Drawing for the job (mm, zero at the part's lowest x, y, z). Coordinates: 2 decimals unless noted, no trailing zeros. Write each loop counter-clockwise with the first axis right and the second up, starting at its lowest first coordinate (ties: lowest second). Pieces come first, ordered by that corner, then holes. Notation, with made-up numbers: M 44.25,13 L 92.25,13 A22 cw 92.25,45 Z; hole C 28.5,23 d9. An arc over 180 degrees is marked long. Put each result on its own line as item: value. Start each with the question number.
Q1. Drop flat-ended pins along their axis: pin 1 (5 mm diameter, centred on x = 25, y = 4.5, fed in from +Z); pin 2 (3 mm diameter, centred on x = 41, y = 6.5, fed in from -Z); pin 3 (3 mm diameter, centred on y = 4.5, z = 2, fed in from +X). Give the stop position or say it passes through.
Q2. Cut at D-D (x = 19.5). Write the cut outline in (y, z), then the cut area to 3 significant figures.
Q3. Cut at A-A (x = 37.5). Write the cut outline in (y, z), then the cut area to 3 significant figures.
Q4. Cut at C-C (z = 0.5). Write the cut outline in (x, y).
Q5. Drill centre lines: line 1 along X through (y, z) = (3, 3.25); line 2 along Z through (x, y) = (33.5, 9.75); line 3 along X through (y, z) = (9.25, 6). Where is each one in solid material? Low to high.
Q6. Cut at B-B (y = 9). Write the cut outline in (x, z).
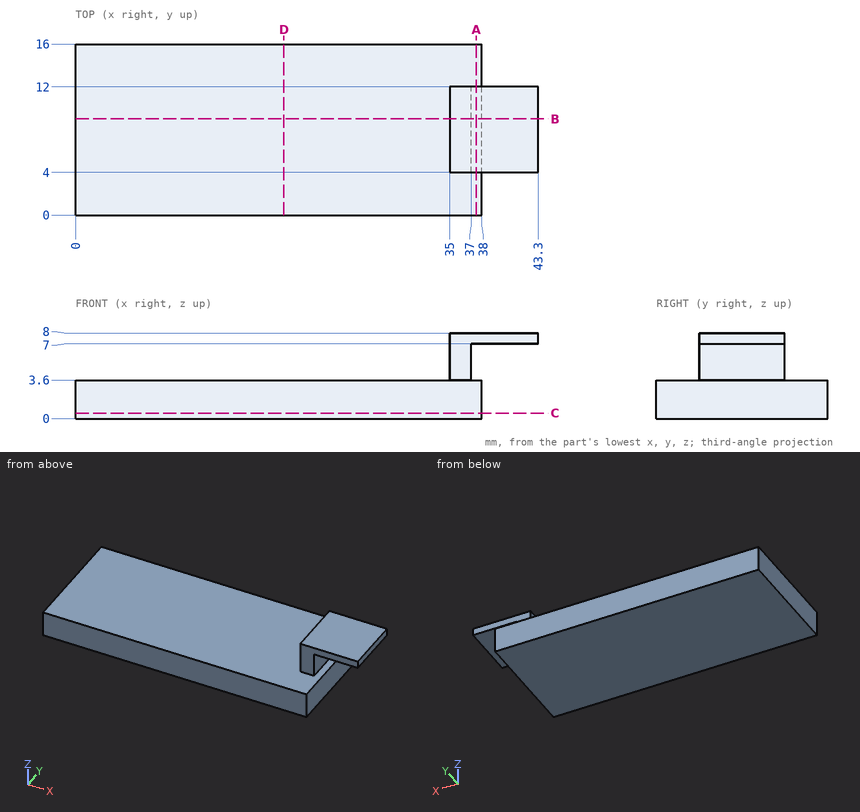
Computed values:
1. pin 1: z = 3.6
1. pin 2: z = 7
1. pin 3: x = 38
2. outline: M 0,0 L 16,0 L 16,3.6 L 0,3.6 Z
2. area: 57.6 mm2
3. outline: M 0,0 L 16,0 L 16,3.6 L 0,3.6 Z; M 4,7 L 12,7 L 12,8 L 4,8 Z
3. area: 65.6 mm2
4. outline: M 0,0 L 38,0 L 38,16 L 0,16 Z
5. line 1: 0 to 38
5. line 2: 0 to 3.6
5. line 3: 35 to 37
6. outline: M 0,0 L 38,0 L 38,3.6 L 37,3.6 L 37,7 L 43.3,7 L 43.3,8 L 35,8 L 35,3.6 L 0,3.6 Z
